Here's how the part is built. I have some questions about the finished solid (model axes, mm). Face numbers are marked on the shaded views. A direction names the side the tool comes from. Coordinates: 2 decimals unless noted, no trailing zeros. Write each loop counter-clockwise with the first axis right and the second up, starting at its lowest first coordinate (ties: lowest second). Pieces come first, ordered by that corner, then holes. Notation, with made-up numbers: M -26,67.25 L -17,67.25 A28 cw -17,85.25 Z; hole C -30.5,38.5 d3. An arc over 180 degrees is marked long. Use one line per item in the form item = value. Start each with the question number.
1. I'm going to push a flat-ended pin straight in: pin 1 Ø0.6 at (y, z) = (0, 1.5) entering from -X. Where does the tip first touch, or does it pass through?
2. On a 3-axis mill with a long thin cutter (end or side, diameter ignored), from which of +Z, -Z, +X, -X, +Y, -Y can I reach the whole of each face in a straight line? I mean the marked faces 1 and 2. Say none if no direction works.
3. Please list where these lines run through material, in increasing order: line 1 along Z through (x, y) = (-0.3, -0.7); line 2 along Y through (x, z) = (0.55, 1); line 3 along X through (y, z) = (-0.05, -6.25). Write a range as [from, to].
4. I want a section at A-A, the plane z = -5.75. List the corners of the cut face in (x, y) for me.
from build123d import *

# Parameters (mm, degrees)
CUT_EXTRUDE1_DEPTH = 1.524


with BuildPart() as part:
    # Sketch1 → Revolve1 (revolve)
    with BuildSketch(Plane(origin=(0, 0, 0), x_dir=(0, 0, -1), z_dir=(1, 0, 0))):
        with BuildLine():
            Line((-1.905, 0), (-1.905, 0.508))
            ThreePointArc((-1.905, 0.508), (-1.533025612, 1.406025612), (-0.635, 1.778))
            Line((-0.635, 1.778), (-0.250000008, 1.778))
            ThreePointArc((-0.250000008, 1.778), (-0.073223307, 1.704776693), (0, 1.527999992))
            Line((0, 1.527999992), (0, 1.25))
            Line((0, 1.25), (7.224, 1.25))
            Line((7.224, 1.25), (7.5, 0.974))
            Line((7.5, 0.974), (7.5, 0))
            Line((7.5, 0), (-1.905, 0))
        make_face()
    revolve(axis=Axis((0, 0, -7.5), (0, 0, 1)))

    # Sketch2 → Cut-Extrude1 (cut)
    with BuildSketch(Plane.XY.offset(0.508)):
        Polygon((-1.25000004, 0.399999962), (-1.25000004, -0.399999962), (-0.594105965, -0.331062717), (-0.421980421, -0.421980421), (-0.331062717, -0.594105965), (-0.399999962, -1.25000004), (0.399999962, -1.25000004), (0.331062717, -0.594105965), (0.421980421, -0.421980421), (0.594105965, -0.331062717), (1.25000004, -0.399999962), (1.25000004, 0.399999962), (0.594105965, 0.331062717), (0.421980421, 0.421980421), (0.331062717, 0.594105965), (0.399999962, 1.25000004), (-0.399999962, 1.25000004), (-0.331062717, 0.594105965), (-0.421980421, 0.421980421), (-0.594105965, 0.331062717), align=None)
    extrude(amount=CUT_EXTRUDE1_DEPTH, mode=Mode.SUBTRACT)


solid = part.part
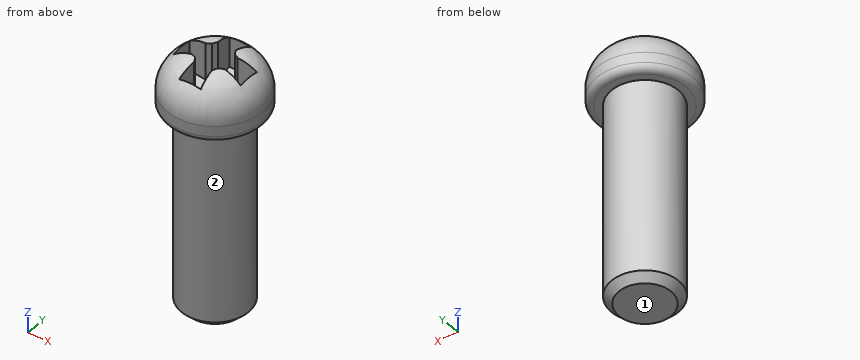
Answer list:
q1.pin_1 = -1.65
q2.face_1 = -Z, +X, -X, +Y, -Y
q2.face_2 = -Z
q3.line_1 = [-7.5, 0.51]
q3.line_2 = [-1.63, -0.35], [0.35, 1.63]
q3.line_3 = [-1.25, 1.25]
q4.outline = C 0,0 d2.5
